The model under review builds one solid part; all positions refer to its coordinate system, in mm. A direction names the side the tool comes from. Coordinates: 2 decimals unless noted, no trailing zeros. Write each loop counter-clockwise with the first axis right and the second up, starting at its lowest first coordinate (ties: lowest second). Pieces come first, ordered by that corner, then holes.
1) Add section B-B, the plane z = 11.5. State the section outline as (x, y) points, then the cut area to 3 significant figures.
2) Add section A-A, the plane y = 32.5. State the section outline as (x, z) points.
3) Mouldability with a two-part tool opening along X and no side actions: class faces 5 (the cylindrical face through (-13.56, 1.45, 19.62)), 6 (the flat face through (-42, 6.73, 20)), 7 (the flat face through (-37.93, 44, 12)) as released by +X, released by -X, zero draft, split by the parting line, or undercut.
4) Add section D-D, the plane x = -35. State the section outline as (y, z) points, then the cut area to 3 significant figures.
5) Add section C-C, the plane y = 21. State the section outline as (x, z) points, then the cut area to 3 significant figures.
6) For P1, Ø2, axis at x = -12.8, z = 20.1, coming from the +Y side; P2, Ø7.5, axis at x = -26, y = 30, coming from the +Z side; P3, Ø3.5, axis at x = -6, z = 18, coming from the +Y side, all flat-tipped, find the tip position at first contact; note any pin that passes through.
7) Machinability: for faces 1 (the flat face through (-14.947, 1, 20)), 2 (the flat face through (-42, 9.562, 20)), 3 (the flat face through (-42, 13.43, 20)), 4 (the flat face through (-44, 37.93, 12)), which of the approach directions +Z, -Z, +X, -X, +Y, -Y give a long, thin tool a straight path to every point of the face, cutting with its end or side? Answer none if there is none.
8) For line 1 (X direction, y = 28.25, z = 20.1); line 2 (Y direction, x = -7, z = 16.25); line 3 (Y direction, x = 2, z = 16.25), list the stretches that pass through material, from the lowest coordinate up.
Autodesk Inventor part; units mm, degrees
ref_plane "Work Plane1" through (0, 0, 10) normal (0, 0, 1) x (1, 0, 0)
ref_plane "Work Plane4" through (-41.8999, 11.7299, 26.2) normal (0, 0, 1) x (1, 0, 0)
ref_plane "YZ Plane" through (0, 0, 0) normal (1, 0, 0) x (0, 1, 0)
ref_plane "Work Plane1" through (0, 0, 10) normal (0, 0, 1) x (1, 0, 0)
sketch "Sketch1" plane through (0, 0, 10) normal (0, 0, 1) x (1, 0, 0)
  line L0 (-4.0299, -0.3538) -> (-2.2322, 1.4439) construction
  arc A0 (-1.4439, 2.2322) -> (-2.2322, 1.4439) centre (-0.9299, 0.9299) ccw construction
  line L1 (-1.4439, 2.2322) -> (0.3538, 4.0299) construction
  line L2 (-37.8299, 42.2137) -> (-37.8299, 45.8299) construction
  line L3 (-37.8299, 45.8299) -> (-4.0299, 45.8299) construction
  line L4 (-4.0299, 45.8299) -> (-4.0299, 42.2137) construction
  line L5 (-4.0299, 4.0299) -> (0.3538, 4.0299)
  circle A1 centre (-20.9299, 20.9299) radius 17.5 construction
  line L6 (-20.9299, 58.9723) -> (17.1124, 20.9299) construction
  line L7 (17.1124, 20.9299) -> (-20.9299, -17.1124) construction
  line L8 (-20.9299, -17.1124) -> (-58.9723, 20.9299) construction
  line L9 (-58.9723, 20.9299) -> (-20.9299, 58.9723) construction
  line L10 (-20.9299, 58.9723) -> (-20.9299, -17.1124) construction
  line L11 (17.1124, 20.9299) -> (-58.9723, 20.9299) construction
  line L12 (-20.9299, 58.9723) -> (32.8701, 58.9723) construction
  line L13 (-43.2198, 43.4299) -> (1.7802, 43.4299) construction
  line L14 (1.7802, 43.4299) -> (1.7802, -1.5701) construction
  line L15 (1.7802, -1.5701) -> (-43.2198, -1.5701) construction
  line L16 (-43.2198, -1.5701) -> (-43.2198, 43.4299) construction
  line L17 (-43.2198, 5.1774) -> (-43.2198, 36.6824)
  line L18 (-43.2198, 36.6824) -> (-36.4723, 43.4299)
  line L19 (-36.4723, 43.4299) -> (-5.3876, 43.4299)
  line L20 (-5.3876, 43.4299) -> (1.7802, 36.2621)
  line L21 (1.7802, 36.2621) -> (1.7802, 5.5977)
  line L22 (1.7802, 5.5977) -> (-5.3876, -1.5701)
  line L23 (-5.3876, -1.5701) -> (-36.4723, -1.5701)
  line L24 (-36.4723, -1.5701) -> (-43.2198, 5.1774)
  line L25 (-4.0299, 42.2137) -> (-37.8299, 42.2137)
  line L26 (-4.0299, -0.3538) -> (-4.0299, 4.0299)
  circle A2 centre (-20.7198, 20.9299) radius 7.0417 construction
  arc A3 (-7.3745, 3.5) -> (-34.4854, 3.5) centre (-20.9299, 0) ccw construction
  arc A4 (-11.4668, 9.7661) -> (-30.4087, 10.1422) centre (-20.7198, 20.9299) ccw
  line L27 (-30.5806, 10.1422) -> (-30.4087, 10.1422)
  line L28 (-30.4087, 10.1422) -> (-30.4087, 1.6029)
  line L29 (-30.4087, 1.6029) -> (-11.4668, 1.6029)
  line L30 (-11.4668, 1.6029) -> (-11.4668, 9.7661)
  line L31 (-43.2198, 43.4299) -> (-10.4667, 10.6769) construction
  line L32 (-8.5595, 8.5517) -> (1.7802, -1.5701) construction
  line L33 (1.7802, 43.4299) -> (-25.699, 15.9507) construction
  line L34 (-30.9728, 10.6769) -> (-43.2198, -1.5701) construction
  point P0 (-37.8299, 4.0299)
  dimension "d18" = 53.8
  dimension "d19" = 45
  dimension "d20" = 53.8
  dimension "d21" = 45
  dimension "d22" = 45
  dimension "d68" = 29
extrude "Extrusion1" add sketch "Sketch1" along normal blind 4 contours L26 L22 L23 L24 L17 L18 L25 L20 L21 L5 | L5 L22 L26 | L25 L18 L19 L20 | L30 L29 L28 A4
sketch "Sketch3" plane through (0, 0, 10) normal (0, 0, -1) x (-1, 0, 0)
  line L0 (37.8299, -0.4701) -> (37.8299, 4.0299) construction
  line L1 (4.0299, 4.0299) -> (4.0299, -0.4701) construction
  line L2 (37.8299, -0.4701) -> (37.8299, 1.1886) construction
  line L3 (4.0299, -3.9701) -> (4.0299, -0.3538) construction
  line L4 (45.8299, 4.0299) -> (42.2137, 4.0299) construction
  line L5 (-0.3538, 4.0299) -> (-3.9701, 4.0299) construction
  line L6 (-3.9701, 37.8299) -> (-0.3538, 37.8299) construction
  line L7 (4.0299, 42.2137) -> (4.0299, 45.8299) construction
  line L8 (37.8299, 45.8299) -> (37.8299, 42.2137) construction
  line L9 (42.2137, 37.8299) -> (45.8299, 37.8299) construction
  line L10 (37.8299, 37.7299) -> (45.8299, 37.7299)
  line L11 (45.8299, 37.7299) -> (45.8299, 4.1299)
  line L12 (45.8299, 4.1299) -> (37.8299, 4.1299)
  line L13 (37.8299, 4.1299) -> (37.8299, 37.7299)
  line L14 (37.7299, 4.0299) -> (4.1299, 4.0299)
  line L15 (4.1299, 4.0299) -> (4.1299, -3.9701)
  line L16 (4.1299, -3.9701) -> (37.7299, -3.9701)
  line L17 (37.7299, -3.9701) -> (37.7299, 4.0299)
  line L18 (4.0299, 4.1299) -> (-3.9701, 4.1299)
  line L19 (-3.9701, 4.1299) -> (-3.9701, 37.7299)
  line L20 (-3.9701, 37.7299) -> (4.0299, 37.7299)
  line L21 (4.0299, 37.7299) -> (4.0299, 4.1299)
  line L22 (4.1299, 37.8299) -> (37.7299, 37.8299)
  line L23 (37.7299, 37.8299) -> (37.7299, 45.8299)
  line L24 (37.7299, 45.8299) -> (4.1299, 45.8299)
  line L25 (4.1299, 45.8299) -> (4.1299, 37.8299)
  point P0 (0, 0)
  dimension "d23" = 0.1
  dimension "d24" = 0.1
  dimension "d25" = 0.1
  dimension "d26" = 0.1
  dimension "d27" = 0.1
extrude "Extrusion3" add sketch "Sketch3" against normal up to surface (4 mm away)
sketch "Skizze12" plane through (0, 0, 10) normal (0, 0, -1) x (-1, 0, 0)
  line L0 (-0.3124, 4.1299) -> (4.1299, -0.3124)
  line L1 (4.1299, -0.3124) -> (4.1299, -3.9701)
  line L2 (4.1299, -3.9701) -> (37.7299, -3.9701) construction
  line L3 (37.7299, -3.9701) -> (37.7299, -0.3124)
  line L4 (37.7299, -0.3124) -> (42.1723, 4.1299)
  line L5 (45.8299, 4.1299) -> (42.1723, 4.1299)
  line L6 (45.8299, 37.7299) -> (45.8299, 4.1299) construction
  line L7 (42.1723, 37.7299) -> (45.8299, 37.7299)
  line L8 (42.1723, 37.7299) -> (37.7299, 42.1723)
  line L9 (37.7299, 42.1723) -> (37.7299, 45.8299)
  line L10 (37.7299, 45.8299) -> (4.1299, 45.8299) construction
  line L11 (4.1299, 45.8299) -> (4.1299, 42.1723)
  line L12 (4.1299, 42.1723) -> (-0.3124, 37.7299)
  line L13 (-3.9701, 37.7299) -> (-0.3124, 37.7299)
  line L14 (-3.9701, 4.1299) -> (-3.9701, 37.7299) construction
  line L15 (-0.3124, 4.1299) -> (-3.9701, 4.1299)
  line L16 (37.9299, -4.1701) -> (3.9299, -4.1701) construction
  line L17 (3.9299, -4.1701) -> (3.9299, -0.3953)
  line L18 (3.9299, -0.3953) -> (-0.3953, 3.9299)
  line L19 (-0.3953, 3.9299) -> (-4.1701, 3.9299)
  line L20 (-4.1701, 3.9299) -> (-4.1701, 37.9299) construction
  line L21 (-4.1701, 37.9299) -> (-0.3953, 37.9299)
  line L22 (-0.3953, 37.9299) -> (3.9299, 42.2551)
  line L23 (3.9299, 42.2551) -> (3.9299, 46.0299)
  line L24 (3.9299, 46.0299) -> (37.9299, 46.0299) construction
  line L25 (37.9299, 46.0299) -> (37.9299, 42.2551)
  line L26 (37.9299, 42.2551) -> (42.2551, 37.9299)
  line L27 (42.2551, 37.9299) -> (46.0299, 37.9299)
  line L28 (46.0299, 37.9299) -> (46.0299, 3.9299) construction
  line L29 (46.0299, 3.9299) -> (42.2551, 3.9299)
  line L30 (42.2551, 3.9299) -> (37.9299, -0.3953)
  line L31 (37.9299, -0.3953) -> (37.9299, -4.1701)
  line L32 (-3.9701, 37.7299) -> (-3.9701, 37.9299)
  line L33 (37.7299, 45.8299) -> (4.1299, 45.8299)
  line L34 (4.1299, 45.8299) -> (3.9299, 45.8299)
  line L35 (37.7299, 45.8299) -> (37.9299, 45.8299)
  line L36 (45.8299, 37.7299) -> (45.8299, 37.9299)
  line L37 (45.8299, 4.1299) -> (45.8299, 3.9299)
  line L38 (37.7299, -3.9701) -> (37.9299, -3.9701)
  line L39 (4.1299, -3.9701) -> (3.9299, -3.9701)
  line L40 (-3.9701, 4.1299) -> (-3.9701, 3.9299)
  point P0 (0, 0)
  dimension "d65" = 0.2
extrude "IM_offset" add sketch "Skizze12" against normal up to surface (4 mm away)
sketch "Sketch15" plane through (0, 0, 14) normal (0, 0, 1) x (1, 0, 0)
  line L0 (-16.2999, 13.4299) -> (-16.2999, 9.2299)
  line L1 (-16.2999, 13.4299) -> (-19.9879, 13.4299)
  line L2 (-21.5499, 13.4299) -> (-19.9879, 13.4299)
  line L3 (-23.112, 13.4299) -> (-21.5499, 13.4299)
  line L4 (-23.112, 13.4299) -> (-37.0999, 13.4299)
  line L5 (-37.0999, 13.4299) -> (-37.0999, 9.2299)
  line L6 (-41.8999, 9.2299) -> (-37.0999, 9.2299)
  line L7 (-41.8999, 9.2299) -> (-41.8999, 6.7299)
  line L8 (-41.8999, 6.7299) -> (-11.4999, 6.7299)
  line L9 (-11.4999, 9.2299) -> (-11.4999, 6.7299)
  line L10 (-16.2999, 9.2299) -> (-11.4999, 9.2299)
  line L11 (3.9701, 37.9299) -> (3.9701, 3.9299)
  line L12 (0.3953, 37.9299) -> (3.9701, 37.9299)
  line L13 (-3.9299, 42.2551) -> (0.3953, 37.9299)
  line L14 (-3.9299, 45.8299) -> (-3.9299, 42.2551)
  line L15 (-37.9299, 45.8299) -> (-3.9299, 45.8299)
  line L16 (-37.9299, 42.2551) -> (-37.9299, 45.8299)
  line L17 (-42.2551, 37.9299) -> (-37.9299, 42.2551)
  line L18 (-45.8299, 37.9299) -> (-42.2551, 37.9299)
  line L19 (-45.8299, 3.9299) -> (-45.8299, 37.9299)
  line L20 (-42.2551, 3.9299) -> (-45.8299, 3.9299)
  line L21 (-37.9299, -0.3953) -> (-42.2551, 3.9299)
  line L22 (-37.9299, -3.9701) -> (-37.9299, -0.3953)
  line L23 (-3.9299, -3.9701) -> (-37.9299, -3.9701)
  line L24 (-3.9299, -0.3953) -> (-3.9299, -3.9701)
  line L25 (0.3953, 3.9299) -> (-3.9299, -0.3953)
  line L26 (3.9701, 3.9299) -> (0.3953, 3.9299)
  line L27 (-45.8299, 3.9299) -> (-38.9491, 3.9299)
  line L28 (-38.9491, 3.9299) -> (-38.9491, 6.7299)
  line L29 (-38.9491, 6.7299) -> (-45.8299, 6.7299)
  line L30 (-45.8299, 6.7299) -> (-45.8299, 3.9299)
  line L31 (3.9701, 3.9299) -> (0.3953, 3.9299)
  line L32 (-14.947, 6.7299) -> (3.9701, 6.7299)
  line L33 (3.9701, 6.7299) -> (3.9701, 3.9299)
  line L34 (3.9701, 3.9299) -> (-14.947, 3.9299)
  line L35 (-14.947, 3.9299) -> (-14.947, 6.7299)
  line L36 (0.3953, 3.9299) -> (-3.9299, -0.3953)
  line L37 (-3.9299, -0.3953) -> (-3.9299, -3.9701)
  line L38 (-3.9299, -3.9701) -> (-37.9299, -3.9701)
  line L39 (-3.9299, -3.9701) -> (-14.947, -3.9701)
  line L40 (-14.947, 3.9299) -> (-14.947, -3.9701)
  line L41 (-45.8299, 3.9299) -> (-45.8299, 37.9299)
  line L42 (-45.8299, 9.5618) -> (-37.5128, 9.5618)
  line L43 (-37.5128, 9.5618) -> (-37.5128, 13.4299)
  line L44 (-37.5128, 13.4299) -> (-45.8299, 13.4299)
  line L45 (-45.8299, 13.4299) -> (-45.8299, 9.5618)
  point P0 (0, 0)
ref_plane "Work Plane4" through (-41.8999, 11.7299, 26.2) normal (0, 0, 1) x (1, 0, 0)
extrude "Extrusion13" add sketch "Sketch15" along normal up to surface (12.2 mm away) contours L32 L11 L26 L34 L35 L8 | L28 L27 L20 L19 L29 L8 | L34 L25 L24 L23 L40 | L19 L44 L43 L42
sketch "Sketch16" plane through (-45.8299, -3.9701, 10) normal (0, -1, 0) x (1, 0, 0)
  circle A0 centre (5.23, 10.1) radius 0.8388
  circle A1 centre (5.23, 10.1) radius 1.5765
  circle A2 centre (33.03, 10.1) radius 2.4
  point P0 (45.8299, -10)
hole "Hole1" at (-40.5999, -3.9701, 20.1) at (-12.7999, -3.9701, 20.1) direction (0, 1, 0) diameter 1.8 end through all
sketch "Sketch17" plane through (0, 0, 14) normal (0, 0, 1) x (1, 0, 0)
  line L0 (-18.1603, 25.8799) -> (-22.3637, 25.8799)
  line L1 (-22.3637, 25.8799) -> (-47.0707, 25.8799)
  line L2 (-19.1999, 18.8799) -> (-19.1999, 25.8799)
  line L3 (-23.8999, 18.8799) -> (-23.8999, 25.8799)
  line L4 (-11.5499, 26.4651) -> (-31.5499, 26.4651)
  line L5 (-31.5499, 26.4651) -> (-31.5499, 33.4651)
  line L6 (-31.5499, 33.4651) -> (-11.5499, 33.4651)
  line L7 (-11.5499, 33.4651) -> (-11.5499, 26.4651)
  point P0 (0, 0)
  dimension "d82" = 20
  dimension "d83" = 7
  dimension "d84" = 7.65
extrude "Extrusion14" add sketch "Sketch17" along normal blind 12
sketch "Sketch18" plane through (-31.5499, 33.4651, 14) normal (0, 1, 0) x (1, 0, 0)
  circle A0 centre (10, -6.1) radius 2.35
  point P0 (31.5499, 14)
extrude "Extrusion15" cut sketch "Sketch18" against normal blind 12
sketch "Sketch19" plane through (0, 0, 26) normal (0, 0, 1) x (1, 0, 0)
  line L0 (-31.5499, 26.4651) -> (-11.5499, 26.4651)
  line L1 (-11.5499, 26.4651) -> (-11.5499, 33.4651)
  line L2 (-11.5499, 33.4651) -> (-31.5499, 33.4651)
  line L3 (-31.5499, 33.4651) -> (-31.5499, 26.4651)
  circle A0 centre (-15.0499, 29.9651) radius 1.45
  circle A1 centre (-28.0499, 29.9651) radius 1.45
  point P0 (0, 0)
  dimension "d89" = 2.9
  dimension "d90" = 3.5
  dimension "d91" = 3.5
  dimension "d92" = 2.9
  dimension "d93" = 3.5
extrude "Extrusion16" cut sketch "Sketch19" against normal through all contours A0 | A1
sketch "Sketch20" plane through (0, 0, 26) normal (0, 0, 1) x (1, 0, 0)
  line L0 (-9.7781, 37.8674) -> (-41.4214, 37.8674)
  line L1 (-41.4214, 37.8674) -> (-41.4214, 22.8936)
  line L2 (-41.4214, 22.8936) -> (-9.7781, 22.8936)
  line L3 (-9.7781, 22.8936) -> (-9.7781, 37.8674)
  point P0 (0, 0)
properties part number "20_Cube_Insert_RaspiCam_v3"
Geometry results:
1. outline: (-45.83, 3.93) - (-42.26, 3.93) - (-37.93, -0.4) - (-37.93, -3.97) - (-3.93, -3.97) - (-3.93, -0.4) - (0.4, 3.93) - (3.97, 3.93) - (3.97, 37.93) - (0.4, 37.93) - (-3.93, 42.26) - (-3.93, 45.83) - (-37.93, 45.83) - (-37.93, 42.26) - (-42.26, 37.93) - (-45.83, 37.93) - close; hole circle Ø2.9 at (-28.05, 29.97); hole circle Ø2.9 at (-15.05, 29.97)
1. area: 2,250 mm2
2. outline: (-45.83, 10) - (3.97, 10) - (3.97, 14) - (-11.55, 14) - (-11.55, 26) - (-31.55, 26) - (-31.55, 14) - (-45.83, 14) - close; hole circle Ø4.7 at (-21.55, 20.1)
3. face 5: undercut
3. face 6: zero draft
3. face 7: released by -X
4. outline: (-3.97, 10) - (45.83, 10) - (45.83, 14) - (-3.97, 14) - close
4. area: 199 mm2
5. outline: (-45.83, 10) - (3.97, 10) - (3.97, 14) - (-45.83, 14) - close
5. area: 199 mm2
6. P1: stops at y = 33.47
6. P2: stops at z = 26
6. P3: stops at y = 6.73
7. face 1: +Z, -Y
7. face 2: +Z, +X, -X
7. face 3: +Z, +X, -X, +Y
7. face 4: +Z, -Z, -X, +Y
8. line 1: x = -31.55 to -23.9, -19.2 to -11.55
8. line 2: y = -3.97 to 6.73
8. line 3: y = 3.93 to 6.73
